Check sheet for the drawn part. Datum: minimum x, y, z corner. Units: mm. Give positions to 0.01 mm unless a question says otherwise; leave off trailing zeros. Loops run counter-clockwise (first coordinate to the right, second up) from the corner with the lowest first, then second, coordinate; pieces in that order, holes last. Notation, with made-up numbers: (-39, 46) - (-4, 46) arc R19 cw to (-4, 71) - close; hole circle Ø1 at (-27, 28). An arc over 180 degrees is marked (long way). Use one line per item in the form item = value.
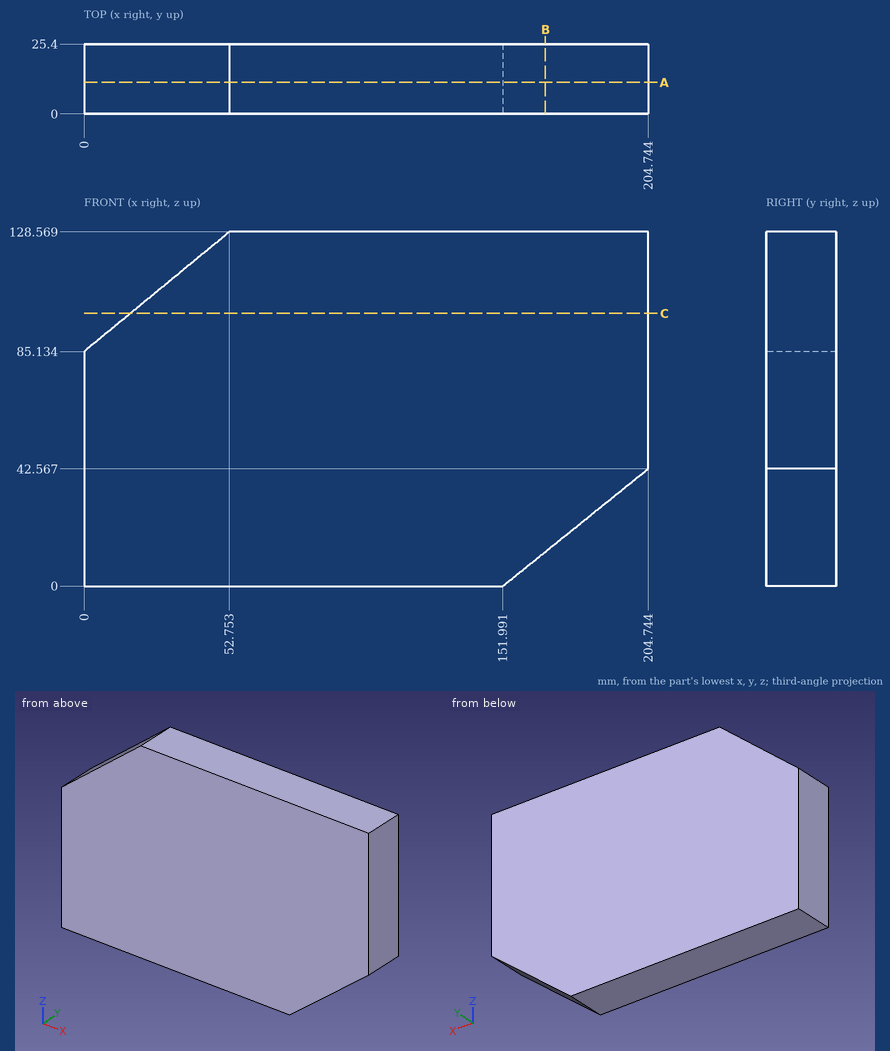
Item 1: Section check A-A on y = 11.5. Record the boundary of the cut face in (x, z).
Answer block:
outline = (0, 0) - (151.99, 0) - (204.74, 42.57) - (204.74, 128.57) - (52.75, 128.57) - (0, 85.13) - close
Item 2: Thickness scan on L1, parallel to Z at x = 46, y = 19.5; L2, parallel to X at y = 12.75, z = 95 (1 decimal); L3, parallel to X at y = 2, z = 42. Record the ranges inside material, lowest first.
Answer block:
L1 = 0 to 123.01
L2 = 12 to 204.7
L3 = 0 to 204.04
Item 3: Section check B-B on x = 167.5. Record the boundary of the cut face in (y, z) (1 decimal).
Answer block:
outline = (0, 12.5) - (25.4, 12.5) - (25.4, 128.6) - (0, 128.6) - close
Item 4: Section check C-C on z = 99. Record the boundary of the cut face in (x, y).
Answer block:
outline = (16.84, 0) - (204.74, 0) - (204.74, 25.4) - (16.84, 25.4) - close
Item 5: Gauge pin test, flat ends, axial feed: P1, Ø6, axis at x = 158, y = 17, coming from the -Z side; P2, Ø1, axis at x = 29, y = 4, coming from the +Z side. Record the tip position at first contact, or that the pin passes through.
Answer block:
P1 = 2.43
P2 = 109.42
